The model under review builds one solid part; all positions refer to its coordinate system, in mm. A direction names the side the tool comes from. Coordinates: 2 decimals unless noted, no trailing zeros. Write each loop counter-clockwise with the first axis right and the second up, starting at its lowest first coordinate (ties: lowest second). Pieces come first, ordered by that corner, then holes.
```python
from build123d import *

# Parameters (mm, degrees)
SKETCH_1_W          = 30
SKETCH_1_H          = 20
SKETCH_1_W_2        = 26
SKETCH_1_H_2        = 16
EXTRUDE_1_DEPTH     = 200
SKETCH_2_R          = 1.6
CUT_EXTRUDE_1_DEPTH = 31
SKETCH_2_3_R        = 3.15
SKETCH_2_3_R_2      = 1.6
CUT_EXTRUDE_2_DEPTH = 3


with BuildPart() as part:
    # Sketch 1 → Extrude 1 (new body)
    with BuildSketch(Plane.XY):
        Rectangle(SKETCH_1_W, SKETCH_1_H)
        Rectangle(SKETCH_1_W_2, SKETCH_1_H_2, mode=Mode.SUBTRACT)
    extrude(amount=EXTRUDE_1_DEPTH)

    # Sketch 2 → Cut-Extrude 1 (cut, through all)
    with BuildSketch(Plane(origin=(15, 0, 0), x_dir=(0, 0, -1), z_dir=(1, 0, 0))):
        with Locations((-58, -4.5)):
            Circle(SKETCH_2_R)
        with Locations((-58, 4.5)):
            Circle(SKETCH_2_R)
        with Locations((-108, 4.5)):
            Circle(SKETCH_2_R)
        with Locations((-108, -4.5)):
            Circle(SKETCH_2_R)
    extrude(amount=-CUT_EXTRUDE_1_DEPTH, mode=Mode.SUBTRACT)

    # Sketch 2_3 → Cut-Extrude 2 (cut)
    with BuildSketch(Plane(origin=(15, 0, 0), x_dir=(0, 0, -1), z_dir=(1, 0, 0))):
        with Locations((-108, -4.5)):
            Circle(SKETCH_2_3_R)
        with Locations((-108, -4.5)):
            Circle(SKETCH_2_3_R_2, mode=Mode.SUBTRACT)
        with Locations((-108, 4.5)):
            Circle(SKETCH_2_3_R)
        with Locations((-108, 4.5)):
            Circle(SKETCH_2_3_R_2, mode=Mode.SUBTRACT)
        with Locations((-58, -4.5)):
            Circle(SKETCH_2_3_R)
        with Locations((-58, -4.5)):
            Circle(SKETCH_2_3_R_2, mode=Mode.SUBTRACT)
        with Locations((-58, 4.5)):
            Circle(SKETCH_2_3_R)
        with Locations((-58, 4.5)):
            Circle(SKETCH_2_3_R_2, mode=Mode.SUBTRACT)
    extrude(amount=-CUT_EXTRUDE_2_DEPTH, mode=Mode.SUBTRACT)


solid = part.part
```
Item 1: Machinability: for faces 1 (the face through (-13.986, 4.981, 56.474)), 2 (the face through (13, 0, 99)), 3 (the face through (14.014, -4.362, 111.147)), which of the approach directions +Z, -Z, +X, -X, +Y, -Y give a long, thin tool a straight path to every point of the face, cutting with its end or side? Answer none if there is none.
Solved:
face 1: +X, -X
face 2: +Z, -Z
face 3: +X
Item 2: Take a section at A-A, the plane x = 4.75. Write out the cut boundary in (y, z).
Solved:
outline: (-10, 0) - (-8, 0) - (-8, 200) - (-10, 200) - close; (8, 0) - (10, 0) - (10, 200) - (8, 200) - close
Item 3: For pin 1 (4 mm diameter, centred on y = -4.5, z = 58, fed in from +X), flat-tipped, find the tip position at first contact; note if it passes through.
Solved:
pin 1: stops at x = -13
Item 4: Take a section at B-B, the plane z = 47.5. Write out the cut boundary in (x, y), plus the area to 3 significant figures.
Solved:
outline: (-15, -10) - (15, -10) - (15, 10) - (-15, 10) - close; hole (-13, -8) - (13, -8) - (13, 8) - (-13, 8) - close
area: 184 mm2
Item 5: To check wall thickness, follow line 1 along Y through (x, z) = (13.6, 108); line 2 along Y through (x, z) = (4.5, 125.5); line 3 along X through (y, z) = (-5.25, 95). State the ranges of each line that lie inside material, in increasing order.
Solved:
line 1: y = -10 to -7.65, -1.35 to 1.35, 7.65 to 10
line 2: y = -10 to -8, 8 to 10
line 3: x = -15 to -13, 13 to 15
Item 6: Mouldability with a two-part tool opening along Y and no side actions: class faces 4 (the face through (0, -8, 99)), 5 (the face through (0, -9, 0)), 6 (the face through (0, 10, 99)), 7 (the face through (14.014, 4.638, 111.147)) as pulls with the +Y half, pulls with the -Y half, needs draft (parallel to the pull), parting line crosses it, or undercut.
Solved:
face 4: undercut
face 5: needs draft
face 6: pulls with the +Y half
face 7: undercut
